Model file for the job. Use its own axes, mm. A direction names the side the tool comes from. Coordinates: 2 decimals unless noted, no trailing zeros. Write each loop counter-clockwise with the first axis right and the second up, starting at its lowest first coordinate (ties: lowest second). Pieces come first, ordered by that corner, then holes. Notation, with made-up numbers: (66, -9.75) - (87, -9.75) arc R25 ccw to (87, 2.25) - close; hole circle Ø4 at (-38.75, 18.5). An arc over 180 degrees is marked (long way). Put each result on its own line as item: value. Start each with the question number.
1. Drill centre lines: L1, parallel to X at y = -10.5, z = 1.75; L2, parallel to Y at x = 8, z = 4; L3, parallel to X at y = 0, z = 0.5. Where is each one in solid material? Low to high. Write a range as from..to.
2. Saw through at D-D, the plane x = -12.5. Write the cut outline in (y, z).
3. Drop flat-ended pins along their axis: P1, Ø3, axis at x = -20.5, y = 12, coming from the -Z side; P2, Ø2, axis at x = -1, z = 5.5, coming from the +Y side; P3, Ø2, axis at x = 25, y = 19.5, coming from the +Z side; P4, Ø16.5, axis at x = 12, y = -12, coming from the +Z side. Give the stop position or say it passes through.
4. Saw through at B-B, the plane y = -25. Write the cut outline in (x, z).
5. Saw through at C-C, the plane x = 25. Write the cut outline in (y, z), plus the area to 3 significant figures.
6. Which spindle directions (+Z, -Z, +X, -X, +Y, -Y) get a long thin tool onto all of the face, cutting with end or side? Do faces 4 (the face through (-1, -22.5, 2)), 5 (the face through (0, 0, 5)), 6 (the face through (-25, -19, 6.5)). Say none if no direction does.
7. Pull direction X, two halves, no side cores. Call faces 1 (the face through (-25, 24, 7)), 2 (the face through (27.5, 0, 2)), 3 (the face through (-25, -25, 10)): released by +X, released by -X, zero draft, split by the parting line, or undercut.
8. Saw through at A-A, the plane z = 4. Write the cut outline in (x, y), plus the area to 3 significant figures.
```python
from build123d import *

# Parameters (mm, degrees)
F0_W     = 55
F0_H     = 55
F1_DEPTH = 5
F2_R     = 1
F3_DEPTH = 5
F4_R     = 1
F5_DEPTH = 1.5


with BuildPart() as f1:
    # F0 (on Top) → F1 (new body)
    with BuildSketch(Plane.XY):
        Rectangle(F0_W, F0_H)
        Polygon((18.964466, -22.5), (-22.5, -22.5), (-22.5, 18.964466), align=None, mode=Mode.SUBTRACT)
        Polygon((22.5, -18.964466), (-18.964466, 22.5), (22.5, 22.5), align=None, mode=Mode.SUBTRACT)
    extrude(amount=F1_DEPTH)

    # F2 (on face) → F3 (join)
    with BuildSketch(Plane.XY.offset(5)):
        with Locations((-25, 25)):
            Circle(F2_R)
        with Locations((25, -25)):
            Circle(F2_R)
        with Locations((25, 25)):
            Circle(F2_R)
        with Locations((-25, -25)):
            Circle(F2_R)
    extrude(amount=F3_DEPTH)

    # F4 (on face) → F5 (join)
    with BuildSketch(Plane.XY.offset(5)):
        with Locations((-25, -19)):
            Circle(F4_R)
        with Locations((25, 19)):
            Circle(F4_R)
    extrude(amount=F5_DEPTH)


solid = f1.part
```
Final values:
1. L1: x = -27.5..-22.5, 6.96..14.04, 22.5..27.5
1. L2: y = -27.5..-22.5, -11.54..-4.46, 22.5..27.5
1. L3: x = -27.5..-22.5, -3.54..3.54, 22.5..27.5
2. outline: (-27.5, 0) - (-22.5, 0) - (-22.5, 5) - (-27.5, 5) - close; (8.96, 0) - (16.04, 0) - (16.04, 5) - (8.96, 5) - close; (22.5, 0) - (27.5, 0) - (27.5, 5) - (22.5, 5) - close
3. P1: passes through
3. P2: stops at y = 27.5
3. P3: stops at z = 6.5
3. P4: stops at z = 5
4. outline: (-27.5, 0) - (27.5, 0) - (27.5, 5) - (26, 5) - (26, 10) - (24, 10) - (24, 5) - (-24, 5) - (-24, 10) - (-26, 10) - (-26, 5) - (-27.5, 5) - close
5. outline: (-27.5, 0) - (27.5, 0) - (27.5, 5) - (26, 5) - (26, 10) - (24, 10) - (24, 5) - (20, 5) - (20, 6.5) - (18, 6.5) - (18, 5) - (-24, 5) - (-24, 10) - (-26, 10) - (-26, 5) - (-27.5, 5) - close
5. area: 298 mm²
6. face 4: +Z, -Z
6. face 5: +Z
6. face 6: +Z, +X, -X
7. face 1: undercut
7. face 2: released by +X
7. face 3: zero draft
8. outline: (-27.5, -27.5) - (27.5, -27.5) - (27.5, 27.5) - (-27.5, 27.5) - close; hole (-22.5, -22.5) - (18.96, -22.5) - (-22.5, 18.96) - close; hole (-18.96, 22.5) - (22.5, -18.96) - (22.5, 22.5) - close
8. area: 1,310 mm²
